Verification items for the finished model (mm, model axes). A direction names the side the tool comes from. Round coordinates to 2 decimals unless told otherwise and drop trailing zeros. Write each loop counter-clockwise with the first axis right and the second up, starting at its lowest first coordinate (ties: lowest second). Pieces come first, ordered by that corner, then holes. Notation, with made-up numbers: M 0.25,-34 L 8.25,-34 A18 ccw 8.25,-15 Z; hole C -4,17 d6. An arc over 180 degrees is marked long. One line per item, written item: value. Start each with the question number.
from build123d import *

# Parameters (mm, degrees)
SKETCH1_R           = 2.5
SKETCH1_R_2         = 6.5
SKETCH1_R_3         = 1.5
BOSS_EXTRUDE1_DEPTH = 3


with BuildPart() as part:
    # Sketch1 → Boss-Extrude1 (new body)
    with BuildSketch(Plane.XY):
        with BuildLine():
            Line((31, 4.5), (26, 4.5))
            Line((26, 4.5), (26, -4.5))
            Line((26, -4.5), (31, -4.5))
            Line((31, -4.5), (31, -14.5))
            ThreePointArc((31, -14.5), (30.121320344, -16.621320344), (28, -17.5))
            Line((28, -17.5), (-28, -17.5))
            ThreePointArc((-28, -17.5), (-30.121320344, -16.621320344), (-31, -14.5))
            Line((-31, -14.5), (-31, 14.5))
            ThreePointArc((-31, 14.5), (-30.121320344, 16.621320344), (-28, 17.5))
            Line((-28, 17.5), (28, 17.5))
            ThreePointArc((28, 17.5), (30.121320344, 16.621320344), (31, 14.5))
            Line((31, 14.5), (31, 4.5))
        make_face()
        with Locations((15, -0.654521384)):
            Circle(SKETCH1_R, mode=Mode.SUBTRACT)
        with Locations((1, 0)):
            Circle(SKETCH1_R_2, mode=Mode.SUBTRACT)
        with Locations((-25, 12.75)):
            Circle(SKETCH1_R_3, mode=Mode.SUBTRACT)
        with Locations((25, 12.75)):
            Circle(SKETCH1_R_3, mode=Mode.SUBTRACT)
        with Locations((25, -12.75)):
            Circle(SKETCH1_R_3, mode=Mode.SUBTRACT)
        with Locations((-25, -12.75)):
            Circle(SKETCH1_R_3, mode=Mode.SUBTRACT)
    extrude(amount=BOSS_EXTRUDE1_DEPTH)


solid = part.part
1) Access from +Z, -Z, +X, -X, +Y, -Y to the whole of each face (thin tool, end or side, straight path). Record for faces 5 (the flat face through (26, 0, 1)), 6 (the cylindrical face through (-26.5, 12.8, 1.5)).
2) Cross-section at B-B (y = -12.75). Record the boundary of the cut face in (x, z).
3) Cross-section at A-A (x = 25). Record the boundary of the cut face in (y, z), then the cut area to 3 significant figures.
4) Cross-section at D-D (z = 2.05). Record the boundary of the cut face in (x, y), then the cut area to 3 significant figures.
5) Cross-section at C-C (x = 1). Record the boundary of the cut face in (y, z).
6) Thickness scan on line 1 (Y direction, x = -24.5, z = 2); line 2 (X direction, y = 14, z = 0.7); line 3 (Y direction, x = 24, z = 0.6). Record the ranges inside material, lowest first.
7) Gauge pin test, flat ends, axial feed: pin 1 Ø11.5 at (x, y) = (1, 0) entering from -Z; pin 2 Ø1.5 at (x, z) = (29.5, 1.5) entering from -Y; pin 3 Ø0.9 at (y, z) = (2, 1) entering from +X. Record the tip position at first contact, or that the pin passes through.
8) Mould release check, pull along Y, two halves, no side actions. Record for faces 1 (the flat face through (29, 4.5, 1)), 2 (the flat face through (-6, 0, 0)), 3 (the flat face through (28, -4.5, 1)), 4 (the cylindrical face through (30.14, -16.6, 1.48)): pulls with the +Y half, pulls with the -Y half, needs draft (parallel to the pull), parting line crosses it, or undercut.
Results below:
1. face 5: +Z, -Z, +X
1. face 6: +Z, -Z
2. outline: M -31,0 L -26.5,0 L -26.5,3 L -31,3 Z; M -23.5,0 L 23.5,0 L 23.5,3 L -23.5,3 Z; M 26.5,0 L 31,0 L 31,3 L 26.5,3 Z
3. outline: M -17.5,0 L -14.25,0 L -14.25,3 L -17.5,3 Z; M -11.25,0 L 11.25,0 L 11.25,3 L -11.25,3 Z; M 14.25,0 L 17.5,0 L 17.5,3 L 14.25,3 Z
3. area: 87.0 mm²
4. outline: M -31,-14.5 A3 ccw -28,-17.5 L 28,-17.5 A3 ccw 31,-14.5 L 31,-4.5 L 26,-4.5 L 26,4.5 L 31,4.5 L 31,14.5 A3 ccw 28,17.5 L -28,17.5 A3 ccw -31,14.5 Z; hole C -25,-12.75 d3; hole C -25,12.75 d3; hole C 1,0 d13; hole C 15,-0.65 d5; hole C 25,-12.75 d3; hole C 25,12.75 d3
4. area: 1,940 mm²
5. outline: M -17.5,0 L -6.5,0 L -6.5,3 L -17.5,3 Z; M 6.5,0 L 17.5,0 L 17.5,3 L 6.5,3 Z
6. line 1: y = -17.5 to -14.16, -11.34 to 11.34, 14.16 to 17.5
6. line 2: x = -31 to -25.83, -24.17 to 24.17, 25.83 to 31
6. line 3: y = -17.5 to -13.87, -11.63 to 11.63, 13.87 to 17.5
7. pin 1: passes through
7. pin 2: stops at y = -17.4
7. pin 3: stops at x = 26
8. face 1: undercut
8. face 2: needs draft
8. face 3: undercut
8. face 4: pulls with the -Y half
